Build history of the part. All positions in model axes, mm. A direction names the side the tool comes from. Round coordinates to 2 decimals unless told otherwise and drop trailing zeros. Order: outer loops, then holes, each group sorted by start corner. A loop starts at its lowest first (then second) coordinate and runs counter-clockwise, first axis right, second up. Notation, with made-up numbers: M 44,66.5 L 53,66.5 A24 cw 53,78.5 Z; hole C 41.5,-24 d9. An arc over 180 degrees is marked long. One line per question, with ' | ' between items. Start each with the question number.
from build123d import *

# Parameters (mm, degrees)
SKETCH_1_R          = 2
EXTRUDE_1_DEPTH     = 10
CUT_EXTRUDE_1_DEPTH = 4.5
FILLET_1_R          = 2


with BuildPart() as part:
    # ｽｹｯﾁ1 → ﾎﾞｽ - 押し出し1 (new body)
    with BuildSketch(Plane(origin=(0, 0, 0), x_dir=(1, 0, 0), z_dir=(0, 1, 0))):
        with BuildLine():
            Line((-11.64685703, -43.466662183), (-18.117333157, -67.61480784))
            ThreePointArc((-18.117333157, -67.61480784), (0, -70), (18.117333157, -67.61480784))
            Line((18.117333157, -67.61480784), (11.64685703, -43.466662183))
            ThreePointArc((11.64685703, -43.466662183), (0, -45), (-11.64685703, -43.466662183))
        make_face()
        with Locations(Location((-6.526309611, -49.572243069, 0), (0, 0, 270))):
            Circle(SKETCH_1_R, mode=Mode.SUBTRACT)
        with Locations(Location((6.526309611, -49.572243069, 0), (0, 0, 90))):
            Circle(SKETCH_1_R, mode=Mode.SUBTRACT)
    extrude(amount=EXTRUDE_1_DEPTH)

    # ｽｹｯﾁ2 → ｶｯﾄ - 押し出し1 (cut)
    with BuildSketch(Plane.XZ):
        with BuildLine():
            Line((14.882095093, 55.540735012), (11.64685703, 43.466662183))
            ThreePointArc((11.64685703, 43.466662183), (0, 45), (-11.64685703, 43.466662183))
            Line((-11.64685703, 43.466662183), (-14.882095093, 55.540735012))
            ThreePointArc((-14.882095093, 55.540735012), (0, 57.5), (14.882095093, 55.540735012))
        make_face()
    extrude(amount=-CUT_EXTRUDE_1_DEPTH, mode=Mode.SUBTRACT)

    # ﾌｨﾚｯﾄ1
    fillet_1_edges = [part.edges().sort_by_distance(p)[0] for p in [
        (-18.117333157, 5, 67.61480784),
        (-11.64685703, 7.25, 43.466662183),
        (11.64685703, 7.25, 43.466662183),
        (18.117333157, 5, 67.61480784),
    ]]
    fillet(fillet_1_edges, radius=FILLET_1_R)


solid = part.part
Item 1: Cut at C-C on y = 4. Write the cut outline in (x, z), then the cut area to 3 significant figures.
Item 2: Cut at B-B on x = -11.5. Write the cut outline in (y, z), then the cut area to 3 significant figures.
Item 3: Tool access for faces 1 (the face through (0, 0, 63)), 2 (the face through (-0.2, 2.2, 57.5)): list every direction of +Z, -Z, +X, -X, +Y, -Y with a clear straight run to the whole face (end or side of a thin tool).
Item 4: Flat gauge pins, fed straight in: pin 1 (1 mm diameter, centred on y = 7, z = 55, fed in from -X); pin 2 (6 mm diameter, centred on x = -8, y = 3, fed in from -Z) (3 decimals); pin 3 (5 mm diameter, centred on x = 13.5, y = 4.5, fed in from +Z); pin 4 (3 mm diameter, centred on x = -6.53, z = 49.57, fed in from +Y). Where does each tip first touch, or does it go through?
Item 5: Cut at A-A on y = 6.75. Write the cut outline in (x, z).
Item 6: Wall check: line 1 along Y through (x, z) = (3, 54.25); line 2 along X through (y, z) = (2.25, 66); line 3 along Z through (x, y) = (-6, 9.5). Give the ranges that are in metal, low to high. Write a range as [from, to].
Item 7: Cut at D-D on z = 56.75. Write the cut outline in (x, y), then the cut area to 3 significant figures.
Item 8: Two-plate mould, pull along X, no slides. Class faces 3 (the face through (15.515, 6.041, 57.903)), 4 (the face through (-5.93, 7.21, 51.48)), 5 (the face through (0, 5, 70)), 6 (the face through (5.926, 7.212, 47.665)): +X half, -X half, draft (parallel to the pull), parting line (faces both ways), or undercut.
Results found:
1) outline: M -17.59,65.65 L -14.88,55.54 A57.5 cw 14.88,55.54 L 17.59,65.65 A2 ccw 16.12,68.12 A70 ccw -16.12,68.12 A2 ccw Z | area: 415 mm^2
2) outline: M 0,56.34 L 4.5,56.34 L 4.5,44.34 L 10,44.34 L 10,69.05 L 0,69.05 Z | area: 193 mm^2
3) face 1: +Z, -Z, +X, -X, -Y | face 2: -Z, -Y
4) pin 1: stops at x = -14.87 | pin 2: stops at z = 43.875 | pin 3: stops at z = 69.13 | pin 4: passes through
5) outline: M -17.59,65.65 L -12.15,45.36 A2 ccw -9.79,43.92 A45 cw 9.79,43.92 A2 ccw 12.15,45.36 L 17.59,65.65 A2 ccw 16.12,68.12 A70 ccw -16.12,68.12 A2 ccw Z; hole C -6.53,49.57 d4; hole C 6.53,49.57 d4
6) line 1: y = [4.5, 10] | line 2: x = [-17.65, 17.65] | line 3: z = [44.6, 47.64], [51.5, 69.74]
7) outline: M -15.21,0 L -9.26,0 L -9.26,4.5 L 9.26,4.5 L 9.26,0 L 15.21,0 L 15.21,10 L -15.21,10 Z | area: 221 mm^2
8) face 3: +X half | face 4: undercut | face 5: parting line | face 6: undercut
